Source: CAD feature listing. Evaluate the final solid. Frame: model axes, mm. A direction names the side the tool comes from. Round coordinates to 2 decimals unless told otherwise and drop trailing zeros. Loops run counter-clockwise (first coordinate to the right, second up) from the corner with the lowest first, then second, coordinate; pieces in that order, holes last. Notation, with made-up numbers: M 41.5,63.5 L 90.5,63.5 A31 cw 90.5,87.5 Z; hole C 21,24.5 d5. An arc over 180 degrees is marked long. Write each question's results on one line, items separated by ' | '. Start each with the question number.
1. Section A-A on y = 2.75. Output: boundary loops of the cut face in (x, z), and give its area (3 significant figures).
2. Section C-C on y = 8. Output: boundary loops of the cut face in (x, z).
3. Section B-B on x = -0.9. Output: boundary loops of the cut face in (y, z).
4. Contact query for flat-ended pins moving along their axis: pin 1 Ø2 at (x, z) = (1, -9.5) entering from +Y; pin 2 Ø1.2 at (x, y) = (-0.5, -0.5) entering from +Z. Output: stop coordinate, or through.
5. Ray query, line 1 (Z direction, x = 0.6, y = 0.5); line 2 (Z direction, x = 1.3, y = 5); line 3 (Y direction, x = -0.45, z = 15). Return the intervals inside material, ascending.
6. Set-up query: faces 4 (the flat face through (0, 3.5, 28)), 5 (the flat face through (0, 3.5, -28)), 6 (the conical face through (-2.286, -3.199, 24.225)), 7 (the flat face through (0, 4, -22)), 8 (the flat face through (-2.203, 8.962, 22.549)). Return all of +Z, -Z, +X, -X, +Y, -Y with unobstructed straight access to the full face (end or side cutting, diameter ignored); none if empty.
7. Section D-D on z = 15. Output: boundary loops of the cut face in (x, y).
8. Draft query along Z for faces 1 (the flat face through (-2.203, 8.951, -22.538)), 2 (the flat face through (0, 9.5, 27)), 3 (the conical face through (-2.286, -3.225, -24.199)). Return one class per face: released by +Z, released by -Z, zero draft, split by the parting line, or undercut.
Autodesk Inventor part; units mm, degrees
ref_plane "YZ Plane" through (0, 0, 0) normal (1, 0, 0) x (0, 1, 0)
ref_plane "XZ Plane" through (0, 0, 0) normal (0, 1, 0) x (-1, 0, 0)
ref_plane "XY Plane" through (0, 0, 0) normal (0, 0, 1) x (1, 0, 0)
sketch "スケッチ1" plane through (0, 0, 0) normal (1, 0, 0) x (0, 1, 0)
  line L0 (-6.7, 0) -> (12.2, 0)
  line L1 (0, 43.4) -> (0, -43.4)
  line L2 (0, 22) -> (0, -22)
  line L3 (0, -22) -> (9.5, -22)
  line L4 (9.5, -22) -> (9.5, -31)
  line L5 (9.5, -31) -> (3.5, -31)
  line L6 (3.5, -31) -> (3.5, -25)
  line L7 (3.5, -25) -> (-4, -25)
  line L8 (-4, -25) -> (-4, 25)
  line L9 (-4, 25) -> (3.5, 25)
  line L10 (3.5, 25) -> (3.5, 31)
  line L11 (3.5, 31) -> (9.5, 31)
  line L12 (9.5, 31) -> (9.5, 22)
  line L13 (9.5, 22) -> (0, 22)
  point P0 (0, 0)
  dimension "d0" = 3.5
  dimension "d1" = 4
  dimension "d2" = 50
  dimension "d3" = 6
  dimension "d4" = 3
  dimension "d5" = 6
extrude "押し出し1" add sketch "スケッチ1" along normal mid plane 4.8
chamfer "面取り1" distance 0.8 angle 45 10 edges at (0, 9.5, 31) (0, 3.5, 31) (2.4, 6.5, 31) (-2.4, 6.5, 31) (2.4, 6.5, -31) (0, 9.5, -31) (-2.4, 6.5, -31) (0, 3.5, -31) (0, 9.5, 22) (0, 9.5, -22)
fillet "フィレット1" radius 2 2 edges at (0, -4, 25) (0, -4, -25)
chamfer "面取り2" distance 0.4 angle 45 28 edges at (2.4, -4, 0) (2.4, -3.4142, -24.4142) (2.4, 0.75, -25) (2.4, 3.5, -27.6) (2.4, -3.4142, 24.4142) (2.4, 0.75, 25) (2.4, 3.5, 27.6) (-2.4, 0.75, 25) (-2.4, -3.4142, 24.4142) (-2.4, 3.5, 27.6) (-2.4, -4, 0) (-2.4, -3.4142, -24.4142) (-2.4, 0.75, -25) (-2.4, 3.5, -27.6) (2.4, 0, 0) (-2.4, 0, 0) (2.4, 4.35, -22) (2.4, 9.1, -22.4) (2.4, 9.5, -26.5) (-2.4, 9.5, -26.5) (-2.4, 9.1, -22.4) (-2.4, 4.35, -22) (-2.4, 4.35, 22) (-2.4, 9.1, 22.4) (-2.4, 9.5, 26.5) (2.4, 9.5, 26.5) (2.4, 9.1, 22.4) (2.4, 4.35, 22)
properties part number "TrussCC_S1" material "ABS プラスチック"
Taken from the geometry:
1) outline: M -2.4,-24.6 L -2,-25 L 2,-25 L 2.4,-24.6 L 2.4,-22.4 L 2,-22 L -2,-22 L -2.4,-22.4 Z; M -2.4,22.4 L -2,22 L 2,22 L 2.4,22.4 L 2.4,24.6 L 2,25 L -2,25 L -2.4,24.6 Z | area: 28.2 mm^2
2) outline: M -2.4,-30.2 L -1.6,-31 L 1.6,-31 L 2.4,-30.2 L 2.4,-22.4 L 2,-22 L -2,-22 L -2.4,-22.4 Z; M -2.4,22.4 L -2,22 L 2,22 L 2.4,22.4 L 2.4,30.2 L 1.6,31 L -1.6,31 L -2.4,30.2 Z
3) outline: M -4,-23 A2 ccw -2,-25 L 3.5,-25 L 3.5,-30.2 L 4.3,-31 L 8.7,-31 L 9.5,-30.2 L 9.5,-22.8 L 8.7,-22 L 0,-22 L 0,22 L 8.7,22 L 9.5,22.8 L 9.5,30.2 L 8.7,31 L 4.3,31 L 3.5,30.2 L 3.5,25 L -2,25 A2 ccw -4,23 Z
4) pin 1: y = 0 | pin 2: z = 25
5) line 1: -25 to -22, 22 to 25 | line 2: -31 to -22, 22 to 31 | line 3: -4 to 0
6) face 4: +Z, +X, -X, -Y | face 5: -Z, +X, -X, -Y | face 6: +Z, -X, -Y | face 7: +X, -X, +Y | face 8: -X, +Y
7) outline: M -2.4,-3.6 L -2,-4 L 2,-4 L 2.4,-3.6 L 2.4,-0.4 L 2,0 L -2,0 L -2.4,-0.4 Z
8) face 1: undercut | face 2: zero draft | face 3: released by -Z
